```python
from build123d import *

# Parameters (mm, degrees)
F0_W     = 200
F0_H     = 300
F1_DEPTH = 200
F3_DEPTH = 200
F4_R     = 100
F5_DEPTH = 50
F7_DEPTH = 200
F9_DEPTH = 50


with BuildPart() as f1:
    # F0 (on Right) → F1 (new body)
    with BuildSketch(Plane.YZ):
        with Locations((100, 150)):
            Rectangle(F0_W, F0_H)
    extrude(amount=F1_DEPTH)

    # F2 (on Right) → F3 (join)
    with BuildSketch(Plane.YZ):
        Polygon((-200, 0), (0, 0), (0, 300), align=None)
    extrude(amount=F3_DEPTH)

    # F4 (on face) → F5 (join)
    with BuildSketch(Plane.XY.offset(300)):
        with Locations((100, 100)):
            Circle(F4_R)
    extrude(amount=F5_DEPTH)

    # F6 (on Front) → F7 (join)
    with BuildSketch(Plane.XZ):
        Polygon((-200, 0), (0, 0), (0, 300), align=None)
    extrude(amount=-F7_DEPTH)

    # F8 (on face) → F9 (join)
    with BuildSketch(Plane(origin=(0, 200, 0), x_dir=(-1, 0, 0), z_dir=(0, 1, 0))):
        Polygon((-100, 300), (-200, 300), (-200, 0), (0, 0), (0, 300), align=None)
    extrude(amount=F9_DEPTH)


solid = f1.part
```
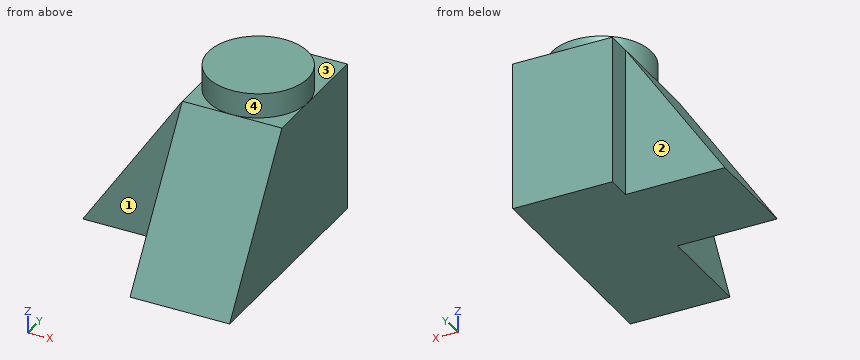
Input: part model. Units: mm. Frame: model coordinates. Face numbers are marked on the shaded views. A direction names the side the tool comes from. Coordinates: 2 decimals unless noted, no trailing zeros. Loops run counter-clockwise (first coordinate to the right, second up) from the corner with the lowest first, then second, coordinate; pieces in that order, holes last. Notation, with made-up numbers: M 63.25,-22.75 L 115.25,-22.75 A26 cw 115.25,2.25 Z; hole C 12.5,57 d3. An arc over 180 degrees is marked long. One line per item, written item: value.
(1) Section C-C (z = 34). Output: boundary loops of the cut face in (x, y).
Filled in:
outline: M -177.33,0 L 0,0 L 0,-177.33 L 200,-177.33 L 200,250 L 0,250 L 0,200 L -177.33,200 Z
(2) Section A-A (y = 16). Output: boundary loops of the cut face in (x, z).
Filled in:
outline: M -200,0 L 200,0 L 200,300 L 154.26,300 L 154.26,350 L 45.74,350 L 45.74,300 L 0,300 Z
(3) Section D-D (y = -37). Output: boundary loops of the cut face in (x, z).
Filled in:
outline: M 0,0 L 200,0 L 200,244.5 L 0,244.5 Z
(4) Reachability of the marked faces 1, 2, 3 and 4 from +Z, -Z, +X, -X, +Y, -Y: full face, straight path, thin tool, end or side. Return the list, or none.
Filled in:
face 1: +Z, -Z, -X, -Y
face 2: +Z, -Z, -X, +Y
face 3: +Z, +Y
face 4: +Z
(5) Line query: line 1 along X through (y, z) = (-107.5, 108.5); line 2 along Z through (x, y) = (179, 205.5). Output: solid intervals per line, ascending. Write a range as from..to.
Filled in:
line 1: 0..200
line 2: 0..300
(6) Pin query (flat end, axial travel): pin 1 (8 mm diameter, centred on x = 110.5, z = 310.5, fed in from -Y); pin 2 (10 mm diameter, centred on x = 148, z = 140.5, fed in from -Y); pin 3 (12 mm diameter, centred on x = -13.5, z = 216.5, fed in from -Y). Return the tip coordinate at first contact, or that it passes through.
Filled in:
pin 1: y = 0.21
pin 2: y = -109.67
pin 3: y = 0
(7) Section B-B (x = -121). Output: boundary loops of the cut face in (y, z), and give its area (3 significant figures).
Filled in:
outline: M 0,0 L 200,0 L 200,118.5 L 0,118.5 Z
area: 23,700 mm^2
